```python
from build123d import *

# Parameters (mm, degrees)
SKIZZE1_R                       = 2
AUFSATZ_LINEAR_AUSTRAGEN1_DEPTH = 1.5
SKIZZE2_R                       = 1
AUFSATZ_LINEAR_AUSTRAGEN2_DEPTH = 9
VERRUNDUNG1_R                   = 1
VERRUNDUNG2_R                   = 0.5
SKIZZE3_W                       = 0.829527345
SKIZZE3_H                       = 0.629507901
SKIZZE3_W_2                     = 0.632202029
SKIZZE3_H_2                     = 0.871689933
SKIZZE3_W_3                     = 0.872489972
SKIZZE3_H_3                     = 0.858509012
SCHNITT_LINEAR_AUSTRAGEN1_DEPTH = 0.5


with BuildPart() as part:
    # Skizze1 → Aufsatz-Linear austragen1 (new body)
    with BuildSketch(Plane.XY):
        Circle(SKIZZE1_R)
    extrude(amount=AUFSATZ_LINEAR_AUSTRAGEN1_DEPTH)

    # Skizze2 → Aufsatz-Linear austragen2 (add)
    with BuildSketch(Plane.XY.offset(1.5)):
        Circle(SKIZZE2_R)
    extrude(amount=AUFSATZ_LINEAR_AUSTRAGEN2_DEPTH)

    # Verrundung1
    verrundung1_edges = [part.edges().sort_by_distance(p)[0] for p in [
        (-1, 0, 10.5),
    ]]
    fillet(verrundung1_edges, radius=VERRUNDUNG1_R)

    # Verrundung2
    verrundung2_edges = [part.edges().sort_by_distance(p)[0] for p in [
        (-2, 0, 0),
    ]]
    fillet(verrundung2_edges, radius=VERRUNDUNG2_R)

    # Skizze3 → Schnitt-Linear austragen1 (cut)
    with BuildSketch(Plane(origin=(0, 0, 0), x_dir=(-1, 0, 0), z_dir=(0, 0, -1))):
        with Locations((-0.731284278, -0.043253269)):
            Rectangle(SKIZZE3_W, SKIZZE3_H)
        with Locations((-0.00041959, 0.707345648)):
            Rectangle(SKIZZE3_W_2, SKIZZE3_H_2)
        with Locations((0.75192641, -0.043253269)):
            Rectangle(SKIZZE3_W_3, SKIZZE3_H)
        with Locations((-0.00041959, -0.787261726)):
            Rectangle(SKIZZE3_W_2, SKIZZE3_H_3)
        with Locations((-0.00041959, -0.043253269)):
            Rectangle(SKIZZE3_W_2, SKIZZE3_H)
    extrude(amount=-SCHNITT_LINEAR_AUSTRAGEN1_DEPTH, mode=Mode.SUBTRACT)


solid = part.part
```
Source: CAD feature listing. Evaluate the final solid. Frame: model axes, mm. A direction names the side the tool comes from. Give positions to 0.01 mm unless a question says otherwise; leave off trailing zeros. Write each loop counter-clockwise with the first axis right and the second up, starting at its lowest first coordinate (ties: lowest second). Pieces come first, ordered by that corner, then holes. Notation, with made-up numbers: (-34, 66.25) - (23, 66.25) arc R19 ccw to (23, 85.25) - close; hole circle Ø5 at (86, 81). An arc over 180 degrees is marked (long way). One line per item, written item: value. Start each with the question number.
Q1. Draft query along X for faces 3 (the face through (0, 0, 0.5)), 4 (the face through (0, -1, 5)), 5 (the face through (0.6, -0.6, 0)). Return one class per face: +X half, -X half, draft (parallel to the pull), parting line (faces both ways), or undercut.
Q2. Set-up query: faces 1 (the face through (0, -2, 1)), 2 (the face through (1, -1, 1.5)). Return all of +Z, -Z, +X, -X, +Y, -Y with unobstructed straight access to the full face (end or side cutting, diameter ignored); none if empty.
Q3. Section query B-B, the plane x = 0. Return the cut outline in (y, z), then the cut area to 3 significant figures.
Q4. Section query A-A, the plane y = 0. Return the cut outline in (x, z).
Q5. Section query D-D, the plane z = 9.75. Return the cut outline in (x, y).
Q6. Material intervals for probe 1 along Z at (x, y) = (-0.3, 1.4); probe 2 along Y at (x, z) = (0, 2), sorted ascending. Write a range as from..to.
Q7. First-contact query: pin 1 Ø1.5 at (y, z) = (0.5, 9) entering from +X; pin 2 Ø0.6 at (x, z) = (0, 0) entering from -Y; pin 3 Ø0.6 at (y, z) = (-1, 0) entering from +X. Flat tips, straight axial feed; report the tip coordinate or a pass-through.
Q8. Section query C-C, the plane z = 8.25. Return the cut outline in (x, y), then the cut area to 3 significant figures.
Answer:
1. face 3: undercut
1. face 4: parting line
1. face 5: draft
2. face 1: +Z, -Z
2. face 2: +Z
3. outline: (-2, 0.5) arc R0.5 ccw to (-1.5, 0) - (-1.22, 0) - (-1.22, 0.5) - (1.14, 0.5) - (1.14, 0) - (1.5, 0) arc R0.5 ccw to (2, 0.5) - (2, 1.5) - (1, 1.5) - (1, 9.5) arc R1 ccw to (-1, 9.5) - (-1, 1.5) - (-2, 1.5) - close
3. area: 22.3 mm2
4. outline: (-2, 0.5) arc R0.5 ccw to (-1.5, 0) - (-1.19, 0) - (-1.19, 0.5) - (1.15, 0.5) - (1.15, 0) - (1.5, 0) arc R0.5 ccw to (2, 0.5) - (2, 1.5) - (1, 1.5) - (1, 9.5) arc R1 ccw to (-1, 9.5) - (-1, 1.5) - (-2, 1.5) - close
5. outline: circle Ø1.94 at (0, 0)
6. probe 1: z = 0..1.5
6. probe 2: y = -1..1
7. pin 1: stops at x = 1
7. pin 2: stops at y = -1.96
7. pin 3: stops at x = 1.74
8. outline: circle Ø2 at (0, 0)
8. area: 3.14 mm2
